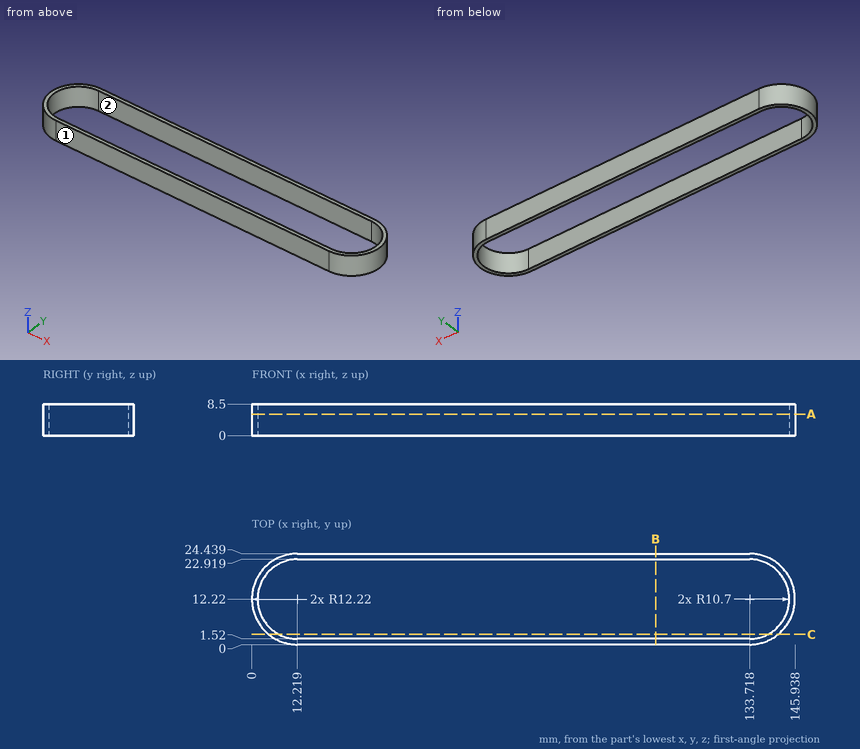
For this review, use the dimensioned drawing (mm, ordinates from the lowest corner) and the shaded views. A direction names the side the tool comes from. Round coordinates to 2 decimals unless told otherwise and drop trailing zeros. Order: outer loops, then holes, each group sorted by start corner. A loop starts at its lowest first (then second) coordinate and runs counter-clockwise, first axis right, second up. Notation, with made-up numbers: M 34.25,29 L 66.25,29 A35 ccw 66.25,62 Z; hole C -2,-21 d3. An arc over 180 degrees is marked long. Use a Markdown table: item, result.
1) Tool access review of the marked faces 1 and 2: name each direction out of +Z, -Z, +X, -X, +Y, -Y from which nothing blocks a thin tool from reaching the whole face with its end or side.
Report:
| item | result |
|---|---|
| face 1 | +Z, -Z, +X, -X, -Y |
| face 2 | +Z, -Z |
2) Insertion check: pin 1 (2 mm diameter, centred on y = 3, z = 1, fed in from -X); pin 2 (1.5 mm diameter, centred on x = 15.5, z = 3.5, fed in from -Y); pin 3 (1.5 mm diameter, centred on y = 7.5, z = 2, fed in from -X). Each pin has a flat end and moves straight along its axis. Give the tip position at first contact, or say it passes through.
Report:
| item | result |
|---|---|
| pin 1 | x = 3.18 |
| pin 2 | y = 0 |
| pin 3 | x = 0.66 |
3) Wall thickness on line 1 along Y through (x, z) = (58.5, 6); line 2 along X through (y, z) = (12, 2.75) (1 decimal); line 3 along X through (y, z) = (9.5, 0.5) (1 decimal): over which ranges is each line inside the solid? List them lowest first. Write a range as [from, to].
Report:
| item | result |
|---|---|
| line 1 | [0, 1.52], [22.92, 24.44] |
| line 2 | [0, 1.5], [144.4, 145.9] |
| line 3 | [0.3, 1.9], [144.1, 145.6] |
4) Consider section C-C (y = 2.75). Write out the cut boundary in (x, z).
Report:
| item | result |
|---|---|
| outline | M 4.5,0 L 7.24,0 L 7.24,8.5 L 4.5,8.5 Z; M 138.7,0 L 141.44,0 L 141.44,8.5 L 138.7,8.5 Z |
5) Consider section A-A (z = 5.75). Write out the cut boundary in (x, y).
Report:
| item | result |
|---|---|
| outline | M 12.22,0 L 133.72,0 A12.22 ccw 133.72,24.44 L 12.22,24.44 A12.22 ccw Z; hole M 12.22,1.52 L 133.72,1.52 A10.7 ccw 133.72,22.92 L 12.22,22.92 A10.7 ccw Z |
6) Consider section B-B (x = 108.5). Write out the cut boundary in (y, z).
Report:
| item | result |
|---|---|
| outline | M 0,0 L 1.52,0 L 1.52,8.5 L 0,8.5 Z; M 22.92,0 L 24.44,0 L 24.44,8.5 L 22.92,8.5 Z |
